Input: part model. Units: mm. Frame: model coordinates. A direction names the side the tool comes from. Coordinates: 2 decimals unless noted, no trailing zeros. Write each loop counter-clockwise with the first axis right and the second up, starting at its lowest first coordinate (ties: lowest second). Pieces come first, ordered by that corner, then holes. Notation, with made-up numbers: M 24.25,58.25 L 67.25,58.25 A17 ccw 67.25,72.25 Z; hole C 21,-23 d3. An arc over 180 degrees is marked long. Answer as a JSON object with one key per item and string values. Group by question number.
from build123d import *

# Parameters (mm, degrees)
F0_W     = 7.62
F0_H     = 31.75
F1_DEPTH = 4.7625
F2_R     = 2.4511
F3_DEPTH = 1.778
F4_W     = 4.572
F4_H     = 28.702
F4_R     = 1.4986
F5_DEPTH = 8.382


with BuildPart() as f1:
    # F0 (on Top) → F1 (new body, symmetric)
    with BuildSketch(Plane.XY):
        Rectangle(F0_W, F0_H)
    extrude(amount=F1_DEPTH, both=True)

    # F2 (on face) → F3 (join)
    with BuildSketch(Plane.XY.offset(4.7625)):
        with Locations((0, 11.9507)):
            Circle(F2_R)
        with Locations((0, 3.9751)):
            Circle(F2_R)
        with Locations((0, -3.9751)):
            Circle(F2_R)
        with Locations((0, -11.9507)):
            Circle(F2_R)
    extrude(amount=F3_DEPTH)

    # F4 (on face) → F5 (cut)
    with BuildSketch(Plane(origin=(0, 0, -4.7625), x_dir=(1, 0, 0), z_dir=(0, 0, -1))):
        Rectangle(F4_W, F4_H)
        with Locations((0, -8.0772)):
            Circle(F4_R, mode=Mode.SUBTRACT)
        Circle(F4_R, mode=Mode.SUBTRACT)
        with Locations((0, 8.0772)):
            Circle(F4_R, mode=Mode.SUBTRACT)
    extrude(amount=-F5_DEPTH, mode=Mode.SUBTRACT)


solid = f1.part
Q1. Section A-A, the plane z = -0.5. Return the cut outline in (x, y) (3 decimals), and give its area (3 significant figures).
Q2. Line query: line 1 (Y direction, x = 0, z = 0.5) (3 decimals); line 2 (X direction, y = 7.5, z = 2.75); line 3 (X direction, y = -2, z = -2.5). Output: solid intervals per line, ascending. Write a range as from..to.
Q3. Draft query along Y for faces 1 (the flat face through (0, 8, -4.762)), 2 (the flat face through (0, -15.875, 0)), 3 (the cylindrical face through (1.43, -0.45, -0.63)). Return one class per face: released by +Y, released by -Y, zero draft, split by the parting line, or undercut.
Q4. Section D-D, the plane y = 3.5. Return the cut outline in (x, z).
Q5. Section B-B, the plane y = 0. Return the cut outline in (x, z).
Q6. Section C-C, the plane z = 5.75. Return the cut outline in (x, y).
Q7. Pin query (flat end, axial travel): pin 1 Ø1 at (x, y) = (-1, 7.5) entering from +Z. Return the tip coordinate at first contact, or that it passes through.
Q8. Access query for faces 4 (the flat face through (0, 0, 4.762)), 5 (the flat face through (0, -14.351, -1)), 6 (the flat face through (3.81, 0, 0)). Directions: +Z, -Z, +X, -X, +Y, -Y. A direction counts if a zero-diameter tool reaches every point of the face in a straight line with its end or side. Return the directions, or none.
Filled in:
{
 "1": {"outline": "M -3.81,-15.875 L 3.81,-15.875 L 3.81,15.875 L -3.81,15.875 Z; C 0,-8.077 d2.997; C 0,0 d2.997; C 0,8.077 d2.997; hole M -2.286,-14.351 L 2.286,-14.351 L 2.286,14.351 L -2.286,14.351 Z", "area": "132 mm^2"},
 "2": {"line 1": "-15.875..-14.351, -9.576..-6.579, -1.499..1.499, 6.579..9.576, 14.351..15.875", "line 2": "-3.81..-2.29, -1.38..1.38, 2.29..3.81", "line 3": "-3.81..-2.29, 2.29..3.81"},
 "3": {"face 1": "zero draft", "face 2": "released by -Y", "face 3": "undercut"},
 "4": {"outline": "M -3.81,-4.76 L -2.29,-4.76 L -2.29,3.62 L 2.29,3.62 L 2.29,-4.76 L 3.81,-4.76 L 3.81,4.76 L 2.4,4.76 L 2.4,6.54 L -2.4,6.54 L -2.4,4.76 L -3.81,4.76 Z"},
 "5": {"outline": "M -3.81,-4.76 L -2.29,-4.76 L -2.29,3.62 L -1.5,3.62 L -1.5,-4.76 L 1.5,-4.76 L 1.5,3.62 L 2.29,3.62 L 2.29,-4.76 L 3.81,-4.76 L 3.81,4.76 L -3.81,4.76 Z"},
 "6": {"outline": "C 0,-11.95 d4.9; C 0,-3.98 d4.9; C 0,3.98 d4.9; C 0,11.95 d4.9"},
 "7": {"pin 1": "z = 4.76"},
 "8": {"face 4": "+Z", "face 5": "-Z", "face 6": "+Z, -Z, +X, +Y, -Y"}
}
